The drawing under review shows one solid part. Ordinate dimensions are in mm from its lowest x, y, z. A direction names the side the tool comes from. Give positions to 0.01 mm unless a question says otherwise; leave off trailing zeros. Loops run counter-clockwise (first coordinate to the right, second up) from the corner with the lowest first, then second, coordinate; pieces in that order, holes last.
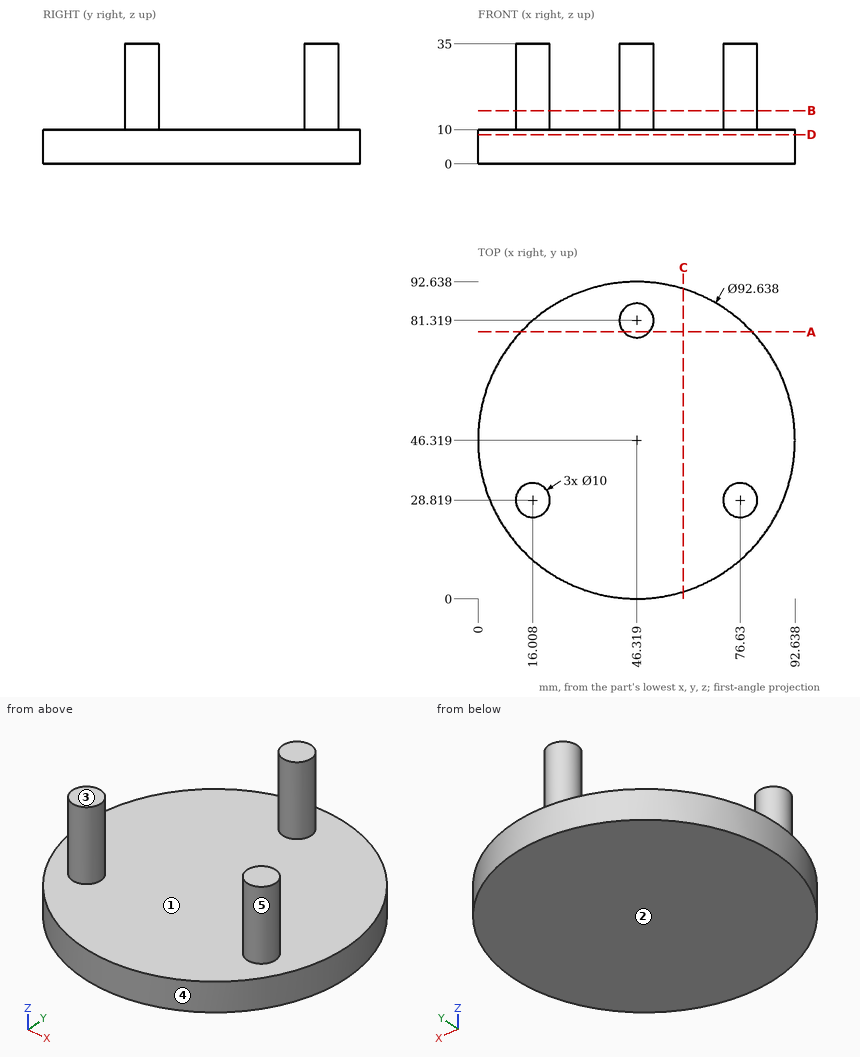
Item 1: Tool access review of the marked faces 1 and 2: name each direction out of +Z, -Z, +X, -X, +Y, -Y from which nothing blocks a thin tool from reaching the whole face with its end or side.
Answer:
face 1: +Z
face 2: -Z, +X, -X, +Y, -Y
Item 2: The part is to be moulded in two halves that separate along X. For the marked faces 3, 4 and 5, say which applies: released by +X, released by -X, zero draft, split by the parting line, or undercut.
Answer:
face 3: zero draft
face 4: split by the parting line
face 5: undercut
Item 3: Take a section at D-D on z = 8.5. Give the boundary of the cut face in (x, y), and give its area (3 significant figures).
Answer:
outline: circle Ø92.64 at (46.32, 46.32)
area: 6,740 mm2
Item 4: Take a section at B-B on z = 15.5. Give the boundary of the cut face in (x, y), and give its area (3 significant figures).
Answer:
outline: circle Ø10 at (16.01, 28.82); circle Ø10 at (46.32, 81.32); circle Ø10 at (76.63, 28.82)
area: 236 mm2
Item 5: Take a section at A-A on y = 78. Give the boundary of the cut face in (x, z), and give its area (3 significant figures).
Answer:
outline: (12.53, 0) - (80.11, 0) - (80.11, 10) - (50.06, 10) - (50.06, 35) - (42.58, 35) - (42.58, 10) - (12.53, 10) - close
area: 863 mm2
Item 6: Take a section at C-C on x = 60. Give the boundary of the cut face in (y, z), and give its area (3 significant figures).
Answer:
outline: (2.07, 0) - (90.57, 0) - (90.57, 10) - (2.07, 10) - close
area: 885 mm2
Item 7: For L1, parallel to Z at x = 65.5, y = 33; L2, parallel to X at y = 26.5, z = 19; L3, parallel to X at y = 28, z = 32 (1 decimal), list the stretches that pass through material, from the lowest coordinate up.
Answer:
L1: z = 0 to 10
L2: x = 11.58 to 20.44, 72.2 to 81.06
L3: x = 11.1 to 20.9, 71.7 to 81.6
Item 8: Clearance check with flat-ended pins moving along their axes: pin 1 Ø4 at (x, z) = (15, 10) entering from +Y; pin 2 Ø1 at (x, y) = (32.5, 67) entering from -Z; pin 3 Ø12 at (x, y) = (39, 48.5) entering from +Z; pin 4 Ø8 at (x, z) = (12.5, 29.5) entering from -Y. State where each tip first meets the part, or that it passes through.
Answer:
pin 1: stops at y = 82.18
pin 2: stops at z = 0
pin 3: stops at z = 10
pin 4: stops at y = 23.82
